Here's how the part is built. I have some questions about the finished solid (model axes, mm). A direction names the side the tool comes from. Coordinates: 2 decimals unless noted, no trailing zeros. Loops run counter-clockwise (first coordinate to the right, second up) from the corner with the lowest first, then second, coordinate; pieces in that order, holes last. Notation, with made-up numbers: (3.25, -9.75) -> (53.25, -9.75) arc R19 ccw to (53.25, 1.25) -> close; hole circle Ø5 at (5.25, 39). An arc over 180 degrees is marked (long way). Answer as a JSON object with one key per item and string values. Group by question number.
Q1. I want a section at C-C on z = -6.25. Write out the boundary of the cut face in (x, y), then the cut area to 3 significant figures.
Q2. I need wall thicknesses on line 1 (Z direction, x = -2, y = 0.5); line 2 (Z direction, x = -1.5, y = 2); line 3 (X direction, y = 0.5, z = -7). Which ranges of each line are inside material? Lowest first, please.
Q3. I want a section at B-B on y = 0. Write out the boundary of the cut face in (x, z), then the cut area to 3 significant figures.
Q4. On a 3-axis mill with a long thin cutter (end or side, diameter ignored), from which of +Z, -Z, +X, -X, +Y, -Y can I reach the whole of each face in a straight line? I mean faces 1 (the cylindrical face through (0, 2, -9)), 2 (the flat face through (0, 0, -14.8)). Say none if no direction works.
Q5. I want a section at A-A on z = -1.25. Write out the boundary of the cut face in (x, y) (3 decimals).
Q6. I'm going to push flat-ended pins straight in: pin 1 (4 mm diameter, centred on y = 3, z = -11.5, fed in from -X); pin 2 (1.5 mm diameter, centred on x = 2, z = -7, fed in from +Y). Where does each tip first touch, or does it pass through?
```python
from build123d import *

# Parameters (mm, degrees)
SKETCH_2_OUTSIDE_W  = 13.726
SKETCH_2_OUTSIDE_H  = 13.726
CUT_EXTRUDE_1_DEPTH = 2.8
CHAMFER_1_SIZE      = 0.4
FILLET_1_R          = 0.4


with BuildPart() as part:
    # Эскиз1 → Повернуть1 (revolve)
    with BuildSketch(Plane(origin=(0, 0, 0), x_dir=(1, 0, 0), z_dir=(0, 1, 0))):
        Polygon((0, 0), (-4, 0), (-4, 2.8), (-2, 2.8), (-2, 14.8), (0, 14.8), align=None)
    revolve(axis=Axis((0, 0, -14.8), (0, 0, 1)))

    # Эскиз2 outside → Вырез-Вытянуть1 (cut)
    with BuildSketch(Plane.XY):
        Rectangle(SKETCH_2_OUTSIDE_W, SKETCH_2_OUTSIDE_H)
        Polygon((0, 3.83), (-3.316877296, 1.915), (-3.316877296, -1.915), (0, -3.83), (3.316877296, -1.915), (3.316877296, 1.915), align=None, mode=Mode.SUBTRACT)
    extrude(amount=-CUT_EXTRUDE_1_DEPTH, mode=Mode.SUBTRACT)

    # Эскиз3 → Вырез-Повернуть1 (revolve, cut)
    with BuildSketch(Plane(origin=(0, 0, 0), x_dir=(0, 0, -1), z_dir=(1, 0, 0))):
        Polygon((0, 3.83), (0.291561886, 3.83), (0, 3.325), align=None)
    revolve(axis=Axis((0, 0, 0), (0, 0, 1)), mode=Mode.SUBTRACT)

    # Фаска1
    chamfer_1_edges = [part.edges().sort_by_distance(p)[0] for p in [
        (2, 0, -14.8),
    ]]
    chamfer(chamfer_1_edges, length=CHAMFER_1_SIZE)

    # Скругление1
    fillet_1_edges = [part.edges().sort_by_distance(p)[0] for p in [
        (2, 0, -2.8),
    ]]
    fillet(fillet_1_edges, radius=FILLET_1_R)


solid = part.part
```
Result set:
{
 "1": {"outline": "circle Ø4 at (0, 0)", "area": "12.6 mm²"},
 "2": {"line 1": "z = -2.99 to 0", "line 2": "z = -2.8 to 0", "line 3": "x = -1.94 to 1.94"},
 "3": {"outline": "(-3.32, -2.8) -> (-2.4, -2.8) arc R0.4 cw to (-2, -3.2) -> (-2, -14.4) -> (-1.6, -14.8) -> (1.6, -14.8) -> (2, -14.4) -> (2, -3.2) arc R0.4 cw to (2.4, -2.8) -> (3.32, -2.8) -> (3.32, 0) -> (-3.32, 0) -> close", "area": "66.5 mm²"},
 "4": {"face 1": "-Z", "face 2": "-Z, +X, -X, +Y, -Y"},
 "5": {"outline": "(-3.317, -1.915) -> (0, -3.83) -> (3.317, -1.915) -> (3.317, 1.915) -> (0, 3.83) -> (-3.317, 1.915) -> close"},
 "6": {"pin 1": "stops at x = -1.73", "pin 2": "stops at y = 1.56"}
}
